Read the model definition and answer for the solid it produces. Units are mm, in the model's axes. A direction names the side the tool comes from. Coordinates: 2 decimals unless noted, no trailing zeros. Order: outer loops, then holes, each group sorted by start corner. A loop starts at its lowest first (then second) coordinate and runs counter-clockwise, first axis right, second up. Notation, with made-up numbers: M 12.5,-32.75 L 16.5,-32.75 A7 cw 16.5,-24.75 Z; hole C -32,-11.5 d4. An arc over 180 degrees is marked long. Use a Markdown table: item, result. Add a question column.
1) For faces 1 (the face through (5, 54.4, 12.3)), 2 (the face through (11.7, 62.3, 4.8)), 3 (the face through (0, 55, 12)), 4 (the face through (0, 40, 14)), 5 (the face through (2, 52, 24)), determine the directions among +Z, -Z, +X, -X, +Y, -Y from which every point of the face is accessible in a straight line to the end or side of a thin tool.
2) Find section C-C on y = 53. Write down the section's boundary in (x, z).
3) Find section B-B on x = 20. Write down the section's boundary in (y, z), plus the area to 4 significant figures.
4) Each of these flat-tipped pins is pushed along its axis until it touches: pin 1 Ø3 at (x, y) = (-10, 5.65) entering from +Z; pin 2 Ø5.5 at (y, z) = (39, 12.5) entering from +X; pin 3 Ø1 at (x, y) = (-1, 21) entering from +Z; pin 4 Ø3 at (y, z) = (55.5, 6.5) entering from -X. Where does it stop, or does it pass through?
5) Find the intervals of material crossed by probe 1 along Y at (x, z) = (-10, 1.35); probe 2 along X at (y, z) = (5.65, 3.7); probe 3 along Z at (x, y) = (-10, 39), in increasing order. Write a range as [from, to].
6) The mould has two halves that part along Y. Classify faces 6 (the face through (-12, 42.3, 12)), 7 (the face through (2.46, 50.61, 15.84)), 8 (the face through (-20, 25.9, 4.8)), 9 (the face through (-12, 37.3, 12)): released by +Y, released by -Y, zero draft, split by the parting line, or undercut.
7) Find section D-D on y = 5.65. Write down the section's boundary in (x, z).
Autodesk Inventor part; units mm, degrees
ref_plane "YZ Plane" through (0, 0, 0) normal (1, 0, 0) x (0, 1, 0)
ref_plane "XZ Plane" through (0, 0, 0) normal (0, 1, 0) x (-1, 0, 0)
ref_plane "XY Plane" through (0, 0, 0) normal (0, 0, 1) x (1, 0, 0)
sketch "Sketch1" plane through (0, 0, 0) normal (0, 0, 1) x (1, 0, 0)
  line L0 (0, 0) -> (30, 0)
  line L1 (30, 0) -> (30, 42.3)
  line L2 (30, 42.3) -> (0, 42.3)
  line L3 (0, 42.3) -> (0, 0)
  line L4 (0, 0.3) -> (0, 42.3)
  line L5 (0, 42.3) -> (42.3, 42.3)
  line L6 (0, 42.3) -> (30, 42.3)
  line L7 (30, 42.3) -> (30, 62.3)
  line L8 (30, 62.3) -> (0, 62.3)
  line L9 (0, 62.3) -> (0, 42.3)
  line L10 (0, 42.3) -> (-20, 42.3)
  line L11 (-20, 42.3) -> (-20, 0)
  line L12 (-20, 0) -> (0, 0)
  line L13 (0, 0) -> (0, 42.3)
  point P0 (10, 52.3)
  point P1 (25, 52.3)
  point P2 (-10, 32.3)
  point P3 (-10, 5.65)
  dimension "d0" = 30
  dimension "d16" = 42.3
  dimension "d21" = 20
  dimension "d22" = 20
  dimension "d49" = 30
  dimension "d50" = 5
  dimension "d69" = 10
  dimension "d70" = 10
  dimension "d71" = 10
extrude "Extrusion2" add sketch "Sketch1" along normal blind 5
hole "Hole3" at (25, 52.3, 0) at (10, 52.3, 0) at (-10, 32.3, 0) at (-10, 5.65, 0) direction (0, 0, 1) diameter 5 depth 8 tip angle 118
sketch "Sketch2" plane through (0, 0, 0) normal (0, 0, -1) x (-1, 0, 0)
  line L0 (20, 0) -> (-30, 0)
  line L1 (-30, 0) -> (-30, 62.3)
  point P0 (0, 0)
  point P1 (-20, 10)
  dimension "d51" = 10
  dimension "d52" = 10
hole "Hole4" at (20, 10, 0) direction (0, 0, 1) diameter 4 depth 8 tip angle 118
sketch "Sketch3" plane through (0, 0, 0) normal (0, 0, -1) x (-1, 0, 0)
  line L0 (-30, 0) -> (-30, 62.3)
  line L1 (20, 0) -> (-30, 0)
  point P0 (0, 0)
  point P1 (-5, 25)
  dimension "d60" = 25
  dimension "d61" = 25
hole "Hole5" at (5, 25, 0) direction (0, 0, 1) diameter 4 depth 8 tip angle 118
sketch "Sketch4" plane through (0, 0, 5) normal (0, 0, 1) x (1, 0, 0)
  line L0 (-20, 42.3) -> (0, 42.3)
  line L1 (0, 42.3) -> (0, 37.3)
  line L2 (0, 37.3) -> (-20, 37.3)
  line L3 (-20, 37.3) -> (-20, 42.3)
  line L4 (30, 62.3) -> (0, 62.3)
  line L5 (0, 42.3) -> (5, 42.3)
  line L6 (5, 42.3) -> (5, 62.3)
  line L7 (5, 62.3) -> (0, 62.3)
  line L8 (0, 62.3) -> (0, 42.3)
  point P0 (0, 0)
  dimension "d72" = 5
  dimension "d73" = 5
extrude "Extrusion3" add sketch "Sketch4" along normal blind 19
sketch "Sketch5" plane through (-20, 37.3, 5) normal (0, -1, 0) x (1, 0, 0)
  line L0 (20, 19) -> (0, 19)
  line L1 (0, -5) -> (0, 19)
  point P0 (20, -5)
  point P1 (10, 9)
  dimension "d76" = 10
  dimension "d77" = 10
hole "Hole6" at (-10, 37.3, 14) direction (0, 1, 0) diameter 5 depth 8 tip angle 118
sketch "Sketch6" plane through (5, 42.3, 5) normal (1, 0, 0) x (0, 0, -1)
  line L0 (-19, 20) -> (-19, 0)
  line L1 (5, 20) -> (-19, 20)
  point P0 (5, -42.3)
  point P1 (-9, 10)
  dimension "d85" = 10
  dimension "d86" = 10
hole "Hole7" at (5, 52.3, 14) direction (-1, 0, 0) diameter 5 depth 8 tip angle 118
properties part number "Corner Mount"
Check result:
| question | item | result |
|---|---|---|
| 1 | face 1 | +Z, +X, +Y, -Y |
| 1 | face 2 | +Z, -Z, +X, -X, +Y |
| 1 | face 3 | +Z, -Z, -X, +Y |
| 1 | face 4 | +Z, +X, -Y |
| 1 | face 5 | +Z, +X, -X, +Y, -Y |
| 2 | outline | M 0,0 L 7.6,0 L 7.6,5 L 5,5 L 5,11.6 L 0,11.6 Z; M 0,16.4 L 5,16.4 L 5,24 L 0,24 Z; M 12.4,0 L 22.6,0 L 22.6,5 L 12.4,5 Z; M 27.4,0 L 30,0 L 30,5 L 27.4,5 Z |
| 3 | outline | M 0,0 L 8,0 L 8,5 L 0,5 Z; M 12,0 L 62.3,0 L 62.3,5 L 12,5 Z |
| 3 | area | 291.5 mm2 |
| 4 | pin 1 | passes through |
| 4 | pin 2 | stops at x = 0 |
| 4 | pin 3 | stops at z = 5 |
| 4 | pin 4 | stops at x = 0 |
| 5 | probe 1 | y = [0, 3.15], [8.15, 29.8], [34.8, 42.3] |
| 5 | probe 2 | x = [-20, -12.5], [-7.5, 30] |
| 5 | probe 3 | z = [0, 11.5], [16.5, 24] |
| 6 | face 6 | released by +Y |
| 6 | face 7 | undercut |
| 6 | face 8 | zero draft |
| 6 | face 9 | released by -Y |
| 7 | outline | M -20,0 L -12.5,0 L -12.5,5 L -20,5 Z; M -7.5,0 L 30,0 L 30,5 L -7.5,5 Z |
